from build123d import *

# Parameters (mm, degrees)
SKETCH1_W           = 8.6
SKETCH1_H           = 4.3
BOSS_EXTRUDE1_DEPTH = 4.7
SKETCH2_W           = 2
SKETCH2_H           = 2
BOSS_EXTRUDE2_DEPTH = 4
SKETCH3_R           = 0.4
BOSS_EXTRUDE3_DEPTH = 1.5


with BuildPart() as part:
    # Sketch1 → Boss-Extrude1 (new body)
    with BuildSketch(Plane(origin=(0, 0, 0), x_dir=(1, 0, 0), z_dir=(0, 1, 0))):
        Rectangle(SKETCH1_W, SKETCH1_H)
    extrude(amount=BOSS_EXTRUDE1_DEPTH)

    # Sketch2 → Boss-Extrude2 (add)
    with BuildSketch(Plane.XY.offset(2.15)):
        with Locations((-1, 2.35)):
            Rectangle(SKETCH2_W, SKETCH2_H)
    extrude(amount=BOSS_EXTRUDE2_DEPTH)

    # Sketch3 → Boss-Extrude3 (add)
    with BuildSketch(Plane.XZ):
        with Locations(Location((-2, 0, 0), (0, 0, 270))):
            Circle(SKETCH3_R)
        with Locations(Location((0, 0, 0), (0, 0, 270))):
            Circle(SKETCH3_R)
        with Locations(Location((2, 0, 0), (0, 0, 270))):
            Circle(SKETCH3_R)
    extrude(amount=BOSS_EXTRUDE3_DEPTH)


solid = part.part
Work out the finished part from the listing and answer in its coordinate system (mm). A direction names the side the tool comes from. Give positions to 0.01 mm unless a question says otherwise; leave off trailing zeros. Order: outer loops, then holes, each group sorted by start corner. A loop starts at its lowest first (then second) coordinate and runs counter-clockwise, first axis right, second up. Notation, with made-up numbers: (-35.75, -36) -> (-19.75, -36) arc R16 ccw to (-19.75, -7) -> close; hole circle Ø1 at (59, -37.75). An arc over 180 degrees is marked (long way). Answer as a JSON object with one key per item and string values. Group by question number.
1. Flat-ended cylindrical pins translate along their axes: pin 1 Ø1 at (x, y) = (0, 4) entering from +Z; pin 2 Ø0.6 at (x, z) = (-1, 4.5) entering from -Y; pin 3 Ø0.6 at (y, z) = (3, 3.5) entering from -X. Find the tip coordinate at first contact, or state that the pin passes through.
2. A tool of negligible diameter and unlimited length cuts with its end or side. For faces 1 (the flat face through (0, 2, 4)), 2 (the flat face through (-1, 1.35, 4)), 3 (the flat face through (-2, 2, 4)), 4 (the flat face through (-4.3, 2, 0)), 5 (the flat face through (-1, 3.35, 4)), from which of +Z, -Z, +X, -X, +Y, -Y can it reach the whole face along a straight path? Write none if from no direction.
3. Section D-D on y = 3.75 is taken. Determine the outline of the cut face in (x, z).
4. Section C-C on y = 3 is taken. Determine the outline of the cut face in (x, z).
5. Consider line 1 along Y through (x, z) = (-2, 2); line 2 along Z through (x, y) = (3.5, 1.25); line 3 along X through (y, z) = (1.5, 5.5). Determine where each line is inside the solid, lowest interval first. Write a range as [from, to].
6. Section B-B on x = 2 is taken. Determine the outline of the cut face in (y, z).
7. Section A-A on z = 0 is taken. Determine the outline of the cut face in (x, y).
Result sheet:
{
 "1": {"pin 1": "stops at z = 2.15", "pin 2": "stops at y = 1.35", "pin 3": "stops at x = -2"},
 "2": {"face 1": "+Z, +X, +Y, -Y", "face 2": "+Z, +X, -X, -Y", "face 3": "+Z, -X, +Y, -Y", "face 4": "+Z, -Z, -X, +Y, -Y", "face 5": "+Z, +X, -X, +Y"},
 "3": {"outline": "(-4.3, -2.15) -> (4.3, -2.15) -> (4.3, 2.15) -> (-4.3, 2.15) -> close"},
 "4": {"outline": "(-4.3, -2.15) -> (4.3, -2.15) -> (4.3, 2.15) -> (0, 2.15) -> (0, 6.15) -> (-2, 6.15) -> (-2, 2.15) -> (-4.3, 2.15) -> close"},
 "5": {"line 1": "y = [0, 4.7]", "line 2": "z = [-2.15, 2.15]", "line 3": "x = [-2, 0]"},
 "6": {"outline": "(-1.5, -0.4) -> (0, -0.4) -> (0, -2.15) -> (4.7, -2.15) -> (4.7, 2.15) -> (0, 2.15) -> (0, 0.4) -> (-1.5, 0.4) -> close"},
 "7": {"outline": "(-4.3, 0) -> (-2.4, 0) -> (-2.4, -1.5) -> (-1.6, -1.5) -> (-1.6, 0) -> (-0.4, 0) -> (-0.4, -1.5) -> (0.4, -1.5) -> (0.4, 0) -> (1.6, 0) -> (1.6, -1.5) -> (2.4, -1.5) -> (2.4, 0) -> (4.3, 0) -> (4.3, 4.7) -> (-4.3, 4.7) -> close"}
}
